The model under review builds one solid part; all positions refer to its coordinate system, in mm. Face numbers are marked on the shaded views. A direction names the side the tool comes from. Round coordinates to 2 decimals unless told otherwise and drop trailing zeros. Order: outer loops, then holes, each group sorted by start corner. A loop starts at its lowest first (then second) coordinate and runs counter-clockwise, first axis right, second up. Notation, with made-up numbers: M -27,60.25 L 13,60.25 A14 cw 13,72.25 Z; hole C 23,21.25 d9. An arc over 180 degrees is marked long. Answer as a JSON object with one key per item and string values. Group by question number.
1. Clearance check with flat-ended pins moving along their axes: P1, Ø2, axis at x = 1, z = 12, coming from the -Y side; P2, Ø5, axis at y = -3.5, z = 45, coming from the +X side; P3, Ø6, axis at y = 4.5, z = 40.5, coming from the -X side. State where each tip first meets the part, or that it passes through.
2. Machinability: for the marked faces 1, 2, 3, 4 and 5, which of the approach directions +Z, -Z, +X, -X, +Y, -Y give a long, thin tool a straight path to every point of the face, cutting with its end or side? Answer none if there is none.
3. Add section B-B on y = 6.75. State the section outline as (x, z) points.
4. To check wall thickness, follow probe 1 along Z at (x, y) = (-5.5, 4.5); probe 2 along Z at (x, y) = (-6.5, -6.5); probe 3 along Z at (x, y) = (1.5, -5.75). State the ranges of each line that lie inside material, in increasing order. Write a range as [from, to].
5. Mouldability with a two-part tool opening along Z and no side actions: class the marked faces 6, 7 and 8 as released by +Z, released by -Z, zero draft, split by the parting line, or undercut.
6. Add section A-A on x = -11.5. State the section outline as (y, z) points, and give its area (3 significant figures).
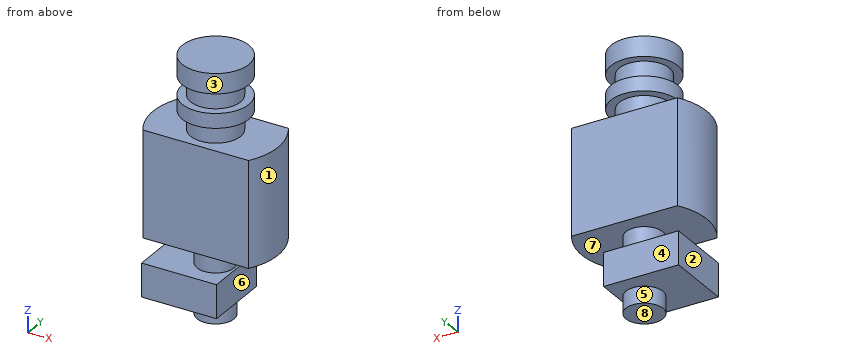
```python
from build123d import *

# Parameters (mm, degrees)
F0_W          = 18
F0_H          = 16
F1_DEPTH      = 8
F2_R          = 4.45
F3_DEPTH      = 14
F3_DEPTH_BACK = 4
F5_DEPTH      = 25.4
F6_R          = 6
F7_DEPTH      = 4.6
F8_R          = 8
F9_DEPTH      = 3.5
F10_R         = 6
F11_DEPTH     = 4.6
F12_R         = 8
F13_DEPTH     = 4.8


with BuildPart() as f1:
    # F0 (on Top) → F1 (new body)
    with BuildSketch(Plane.XY):
        with Locations((-4, 0)):
            Rectangle(F0_W, F0_H)
    extrude(amount=F1_DEPTH)

    # F2 (on Top) → F3 (join, two sides)
    with BuildSketch(Plane.XY) as f3_sk:
        Circle(F2_R)
    extrude(amount=F3_DEPTH)
    extrude(f3_sk.sketch, amount=-F3_DEPTH_BACK)

    # F4 (on face) → F5 (join)
    with BuildSketch(Plane.XY.offset(14)):
        with BuildLine():
            Line((12.6885775404, 8), (-12.6885775404, 8))
            ThreePointArc((-12.6885775404, 8), (-15, 0), (-12.6885775404, -8))
            Line((-12.6885775404, -8), (12.6885775404, -8))
            ThreePointArc((12.6885775404, -8), (15, 0), (12.6885775404, 8))
        make_face()
    extrude(amount=F5_DEPTH)

    # F6 (on face) → F7 (join)
    with BuildSketch(Plane.XY.offset(39.4)):
        Circle(F6_R)
    extrude(amount=F7_DEPTH)

    # F8 (on face) → F9 (join)
    with BuildSketch(Plane.XY.offset(44)):
        Circle(F8_R)
    extrude(amount=F9_DEPTH)

    # F10 (on face) → F11 (join)
    with BuildSketch(Plane.XY.offset(47.5)):
        Circle(F10_R)
    extrude(amount=F11_DEPTH)

    # F12 (on face) → F13 (join)
    with BuildSketch(Plane.XY.offset(52.1)):
        Circle(F12_R)
    extrude(amount=F13_DEPTH)


solid = f1.part
```
Recorded:
{
 "1": {"P1": "stops at y = -4.45", "P2": "stops at x = 7.94", "P3": "stops at x = -14.9"},
 "2": {"face 1": "+Z, -Z, +X", "face 2": "-Z, -X, +Y, -Y", "face 3": "+Z", "face 4": "+Z, -Z, +X, -X, +Y", "face 5": "-Z"},
 "3": {"outline": "M -13.4,14 L 13.4,14 L 13.4,39.4 L -13.4,39.4 Z; M -13,0 L 5,0 L 5,8 L -13,8 Z; M -4.29,44 L 4.29,44 L 4.29,47.5 L -4.29,47.5 Z; M -4.29,52.1 L 4.29,52.1 L 4.29,56.9 L -4.29,56.9 Z"},
 "4": {"probe 1": "z = [0, 8], [14, 39.4], [44, 47.5], [52.1, 56.9]", "probe 2": "z = [0, 8], [14, 39.4]", "probe 3": "z = [0, 8], [14, 56.9]"},
 "5": {"face 6": "zero draft", "face 7": "undercut", "face 8": "released by -Z"},
 "6": {"outline": "M -8,0 L 8,0 L 8,8 L -8,8 Z; M -8,14 L 8,14 L 8,39.4 L -8,39.4 Z", "area": "534 mm²"}
}
